The model under review builds one solid part; all positions refer to its coordinate system, in mm. Coordinates: 2 decimals unless noted, no trailing zeros. Loops run counter-clockwise (first coordinate to the right, second up) from the corner with the lowest first, then second, coordinate; pieces in that order, holes last. Notation, with made-up numbers: M -11.5,10 L 34.5,10 A19 ccw 34.5,26 Z; hole C -9.5,-22.5 d7. An arc over 180 degrees is marked long. Return JSON: item names as keys, results as strings.
```python
from build123d import *

# Parameters (mm, degrees)
F1_DEPTH = 8
F2_R     = 4.99999


# Not quite as in the source:
# - a fillet or chamfer is up to 0.001 mm smaller than in the source, because OpenCascade refuses the exact size


with BuildPart() as f1:
    # F0 (on Front) → F1 (new body)
    with BuildSketch(Plane.XZ):
        with BuildLine():
            ThreePointArc((-36.9956071563, -9.8601329718), (-48.6622738229, 0), (-36.9956071563, 9.8601329718))
            Line((-36.9956071563, 9.8601329718), (-25.9716433602, 7.9967429906))
            ThreePointArc((-25.9716433602, 7.9967429906), (-30.3420228558, 12.4809223955), (-36.1622738229, 14.7901994577))
            ThreePointArc((-36.1622738229, 14.7901994577), (-53.6622738229, 0), (-36.1622738229, -14.7901994577))
            ThreePointArc((-36.1622738229, -14.7901994577), (-30.3420228558, -12.4809223955), (-25.9716433602, -7.9967429906))
            Line((-25.9716433602, -7.9967429906), (-36.9956071563, -9.8601329718))
        make_face()
        with BuildLine():
            ThreePointArc((-36.1622738229, 14.7901994577), (-30.3420228558, 12.4809223955), (-25.9716433602, 7.9967429906))
            Line((-25.9716433602, 7.9967429906), (-9.9451005014, 5.2877628134))
            ThreePointArc((-9.9451005014, 5.2877628134), (-6.064590678, 8.3321209795), (-1.1622738229, 8.8741196746))
            Line((-1.1622738229, 8.8741196746), (-36.1622738229, 14.7901994577))
        make_face()
        with BuildLine():
            Line((-9.9451005014, -5.2877628134), (-25.9716433602, -7.9967429906))
            ThreePointArc((-25.9716433602, -7.9967429906), (-30.3420228558, -12.4809223955), (-36.1622738229, -14.7901994577))
            Line((-36.1622738229, -14.7901994577), (-1.1622738229, -8.8741196746))
            ThreePointArc((-1.1622738229, -8.8741196746), (-6.064590678, -8.3321209795), (-9.9451005014, -5.2877628134))
        make_face()
        with BuildLine():
            ThreePointArc((-1.1622738229, 8.8741196746), (-6.064590678, 8.3321209795), (-9.9451005014, 5.2877628134))
            Line((-9.9451005014, 5.2877628134), (-1.9956071563, 3.9440531887))
            ThreePointArc((-1.9956071563, 3.9440531887), (0.3927766404, 2.5819888975), (1.3377261771, 0))
            ThreePointArc((1.3377261771, 0), (0.3927766404, -2.5819888975), (-1.9956071563, -3.9440531887))
            Line((-1.9956071563, -3.9440531887), (-9.9451005014, -5.2877628134))
            ThreePointArc((-9.9451005014, -5.2877628134), (-6.064590678, -8.3321209795), (-1.1622738229, -8.8741196746))
            ThreePointArc((-1.1622738229, -8.8741196746), (4.2115897195, -5.8094750193), (6.3377261771, 0))
            ThreePointArc((6.3377261771, 0), (4.2115897195, 5.8094750193), (-1.1622738229, 8.8741196746))
        make_face()
    extrude(amount=F1_DEPTH)

    # F2 (radius 5 in the source; OpenCascade refuses exactly that, so slightly less here)
    f2_edges = [f1.edges().sort_by_distance(p)[0] for p in [
        (-18.662274, -8, 11.83216),
    ]]
    fillet(f2_edges, radius=F2_R)


solid = f1.part
```
1. Insertion check: pin 1 Ø1 at (x, z) = (-23, 6) entering from +Y; pin 2 Ø4 at (x, y) = (-3, -3.5) entering from +Z. Each pin has a flat end and moves straight along its axis. Give the tip position at first contact, or say it passes through.
Check values:
{"pin 1": "through", "pin 2": "z = 9.52"}
2. The part is to be moulded in two halves that separate along X. For faces 1 (the face through (-48.66, -3.94, -0.24)), 2 (the face through (-24, 0, 10)), 3 (the face through (-18.907, -1.479, -11.874)), say which applies: released by +X, released by -X, zero draft, split by the parting line, or undercut.
Check values:
{"face 1": "undercut", "face 2": "zero draft", "face 3": "released by +X"}
3. To check wall thickness, follow line 1 (Z direction, x = -31.5, y = -5); line 2 (Z direction, x = -30.5, y = -2.25); line 3 (X direction, y = -7.5, z = 2.75). State the ranges of each line that lie inside material, in increasing order.
Check values:
{"line 1": "-13.58 to -8.93, 8.93 to 13.58", "line 2": "-13.83 to -8.76, 8.76 to 13.83", "line 3": "-50.53 to -48.28, 0.24 to 2.87"}
4. Add section A-A on y = -1.5. Give the boundary of the cut face in (x, z).
Check values:
{"outline": "M -36.16,-14.79 L -1.16,-8.87 A9 ccw -1.16,8.87 L -36.16,14.79 A15 ccw long Z; hole M -37,-9.86 L -2,-3.94 A4 ccw -2,3.94 L -37,9.86 A10 ccw long Z"}
